from build123d import *

# Parameters (mm, degrees)
PAD_DEPTH       = 5
POCKET_DEPTH    = 5
SKETCH002_R     = 1.6
POCKET001_DEPTH = 5
POCKET002_DEPTH = 3
FILLET_R        = 1
SKETCH004_R     = 2.85
POCKET003_DEPTH = 2
CHAMFER_SIZE    = 1.2
SKETCH005_R     = 8.15
POCKET004_DEPTH = 4
SKETCH006_R     = 6.15
POCKET005_DEPTH = 1


with BuildPart() as part:
    # Sketch → Pad (new body)
    with BuildSketch(Plane.XY):
        with BuildLine():
            Line((-35, 70), (35, 70))
            ThreePointArc((55, 50), (49.142136, 64.142136), (35, 70))
            Line((55, 50), (55, 25))
            ThreePointArc((30, 0), (47.67767, 7.32233), (55, 25))
            Line((30, 0), (-30, 0))
            ThreePointArc((-55, 25), (-47.67767, 7.32233), (-30, 0))
            Line((-55, 25), (-55, 50))
            ThreePointArc((-35, 70), (-49.142136, 64.142136), (-55, 50))
        make_face()
    extrude(amount=PAD_DEPTH)

    # Sketch001 (on Face10 of Pad) → Pocket (cut)
    with BuildSketch(Plane.XY.offset(5)):
        with BuildLine():
            Line((-10, 58), (10, 58))
            ThreePointArc((20, 48), (17.071068, 55.071068), (10, 58))
            Line((20, 48), (20, 22))
            ThreePointArc((10, 12), (17.071068, 14.928932), (20, 22))
            Line((10, 12), (-10, 12))
            ThreePointArc((-20, 22), (-17.071068, 14.928932), (-10, 12))
            Line((-20, 22), (-20, 48))
            ThreePointArc((-10, 58), (-17.071068, 55.071068), (-20, 48))
        make_face()
    extrude(amount=-POCKET_DEPTH, mode=Mode.SUBTRACT)

    # Sketch002 (on Face5 of Pocket) → Pocket001 (cut)
    with BuildSketch(Plane.XY.offset(5)):
        with Locations((-51.75, 45)):
            Circle(SKETCH002_R)
        with Locations((-51.75, 30)):
            Circle(SKETCH002_R)
        with Locations((-5, 6)):
            Circle(SKETCH002_R)
        with Locations((5, 6)):
            Circle(SKETCH002_R)
        with Locations((15, 64)):
            Circle(SKETCH002_R)
        with Locations((-15, 64)):
            Circle(SKETCH002_R)
        with Locations((51.75, 45)):
            Circle(SKETCH002_R)
        with Locations((51.75, 30)):
            Circle(SKETCH002_R)
    extrude(amount=-POCKET001_DEPTH, mode=Mode.SUBTRACT)

    # Sketch003 (on Face5 of Pocket001) → Pocket002 (cut)
    with BuildSketch(Plane.XY.offset(5)):
        with BuildLine():
            ThreePointArc((51.75, 48), (48.75, 45), (51.75, 42))
            Line((51.75, 42), (61.75, 42))
            ThreePointArc((61.75, 42), (64.75, 45), (61.75, 48))
            Line((51.75, 48), (61.75, 48))
        make_face()
        with BuildLine():
            ThreePointArc((51.75, 33), (48.75, 30), (51.75, 27))
            Line((51.75, 27), (61.75, 27))
            ThreePointArc((61.75, 27), (64.75, 30), (61.75, 33))
            Line((51.75, 33), (61.75, 33))
        make_face()
        with BuildLine():
            ThreePointArc((-51.75, 42), (-48.75, 45), (-51.75, 48))
            Line((-51.75, 48), (-61.75, 48))
            ThreePointArc((-61.75, 48), (-64.75, 45), (-61.75, 42))
            Line((-51.75, 42), (-61.75, 42))
        make_face()
        with BuildLine():
            ThreePointArc((-51.75, 27), (-48.75, 30), (-51.75, 33))
            Line((-51.75, 33), (-61.75, 33))
            ThreePointArc((-61.75, 33), (-64.75, 30), (-61.75, 27))
            Line((-51.75, 27), (-61.75, 27))
        make_face()
    extrude(amount=-POCKET002_DEPTH, mode=Mode.SUBTRACT)

    # Fillet
    fillet_edges = [part.edges().sort_by_distance(p)[0] for p in [
        (55, 27, 3.5),
        (55, 33, 3.5),
        (55, 42, 3.5),
        (55, 48, 3.5),
        (-55, 48, 3.5),
        (-55, 42, 3.5),
        (-55, 33, 3.5),
        (-55, 27, 3.5),
    ]]
    fillet(fillet_edges, radius=FILLET_R)

    # Sketch004 (on Face6 of Fillet) → Pocket003 (cut)
    with BuildSketch(Plane(origin=(0, 0, 0), x_dir=(1, 0, 0), z_dir=(0, 0, -1))):
        with Locations((-5, -6)):
            Circle(SKETCH004_R)
        with Locations((5, -6)):
            Circle(SKETCH004_R)
        with Locations((-15, -64)):
            Circle(SKETCH004_R)
        with Locations((15, -64)):
            Circle(SKETCH004_R)
    extrude(amount=-POCKET003_DEPTH, mode=Mode.SUBTRACT)

    # Chamfer
    chamfer_edges = [part.edges().sort_by_distance(p)[0] for p in [
        (-6.6, 6, 2),
        (3.4, 6, 2),
        (-16.6, 64, 2),
        (13.4, 64, 2),
    ]]
    chamfer(chamfer_edges, length=CHAMFER_SIZE)

    # Sketch005 (on Face3 of Chamfer) → Pocket004 (cut)
    with BuildSketch(Plane.XY.offset(5)):
        with Locations((-39, 44)):
            Circle(SKETCH005_R)
        with Locations((39, 44)):
            Circle(SKETCH005_R)
    extrude(amount=-POCKET004_DEPTH, mode=Mode.SUBTRACT)

    # Sketch006 (on Face54 of Pocket004) → Pocket005 (cut)
    with BuildSketch(Plane.XY.offset(1)):
        with Locations((-39, 44)):
            Circle(SKETCH006_R)
        with Locations((39, 44)):
            Circle(SKETCH006_R)
    extrude(amount=-POCKET005_DEPTH, mode=Mode.SUBTRACT)


solid = part.part
Input: part model. Units: mm. Frame: model coordinates. A direction names the side the tool comes from. Coordinates: 2 decimals unless noted, no trailing zeros. Order: outer loops, then holes, each group sorted by start corner. A loop starts at its lowest first (then second) coordinate and runs counter-clockwise, first axis right, second up. Notation, with made-up numbers: M -0.75,78 L 47.25,78 A24 ccw 47.25,88 Z; hole C -10,7.5 d8. An arc over 180 degrees is marked long. Write item = value, one per line. Start each with the question number.
(1) First-contact query: P1, Ø5, axis at x = 15, y = 64, coming from the +Z side; P2, Ø2, axis at x = 41, z = 0.5, coming from the +Y side; P3, Ø1.9, axis at x = 51, y = 31.5, coming from the +Z side; P4, Ø0.7, axis at x = -53, z = 3.5, coming from the -Y side. Flat tips, straight axial feed; report the tip coordinate or a pass-through.
(2) Section D-D on x = 42. Output: boundary loops of the cut face in (y, z) (3 decimals).
(3) Section B-B on x = -5. Output: boundary loops of the cut face in (y, z), and give its area (3 significant figures).
(4) Reachability of faces 1 (the flat face through (53, 42, 4)), 2 (the flat face through (-53.31, 29.17, 2)), 3 (the flat face through (35.9, 49.5, 1)), 4 (the flat face through (0, 58, 3)) from +Z, -Z, +X, -X, +Y, -Y: full face, straight path, thin tool, end or side. Return the list, or none.
(5) Pull-direction query (X, two-part tool) for faces 5 (the cylindrical face through (-48.986, 64.297, 2.465)), 6 (the flat face through (20, 35, 3)), 7 (the flat face through (0, 0, 2)), 8 (the cylindrical face through (17.15, 54.99, 2.54)); classes: released by +X, released by -X, zero draft, split by the parting line, or undercut.
(6) Section A-A on y = 30. Output: boundary loops of the cut face in (x, z).
(7) Line query: line 1 along Y through (x, z) = (5, 4.4); line 2 along X through (y, z) = (25.5, 3.3); line 3 along Y through (x, z) = (17, 0.65). Output: solid intervals per line, ascending. Write a range as [from, to].
(8) Section C-C on y = 55. Output: boundary loops of the cut face in (x, z), and give its area (3 significant figures).
Result set:
q1.P1 = 5
q1.P2 = 69.36
q1.P3 = 2
q1.P4 = 14.42
q2.outline = M 3.068,0 L 38.631,0 L 38.631,1 L 36.422,1 L 36.422,5 L 3.068,5 Z; M 49.369,0 L 68.735,0 L 68.735,5 L 51.578,5 L 51.578,1 L 49.369,1 Z
q3.outline = M 0,0 L 3.15,0 L 3.15,2 L 3.2,2 L 4.4,3.2 L 4.4,5 L 0,5 Z; M 7.6,3.2 L 8.8,2 L 8.85,2 L 8.85,0 L 12,0 L 12,5 L 7.6,5 Z; M 58,0 L 70,0 L 70,5 L 58,5 Z
q3.area = 97.6 mm²
q4.face_1 = +Z, +X
q4.face_2 = +Z, -X
q4.face_3 = +Z
q4.face_4 = +Z, -Z
q5.face_5 = released by -X
q5.face_6 = undercut
q5.face_7 = zero draft
q5.face_8 = undercut
q6.outline = M -55,0 L -53.35,0 L -53.35,2 L -55,2 Z; M -50.15,0 L -20,0 L -20,5 L -48.75,5 L -48.75,2 L -50.15,2 Z; M 20,0 L 50.15,0 L 50.15,2 L 48.75,2 L 48.75,5 L 20,5 Z; M 53.35,0 L 55,0 L 55,2 L 53.35,2 Z
q7.line_1 = [0, 4.4], [7.6, 12], [58, 70]
q7.line_2 = [-55, -20], [20, 55]
q7.line_3 = [0, 14.86], [55.14, 61.97], [66.03, 70]
q8.outline = M -54.36,0 L -17.14,0 L -17.14,5 L -54.36,5 Z; M 17.14,0 L 54.36,0 L 54.36,5 L 17.14,5 Z
q8.area = 372 mm²
